Check sheet for the modelled part. Datum: model origin and axes. Units: mm. Face numbers are marked on the shaded views. A direction names the side the tool comes from. Round coordinates to 2 decimals unless told otherwise and drop trailing zeros. Write each loop counter-clockwise with the first axis right and the second up, starting at its lowest first coordinate (ties: lowest second). Pieces come first, ordered by that corner, then holes. Notation, with made-up numbers: (69.5, 4) -> (112.5, 4) arc R25 cw to (112.5, 38) -> close; hole circle Ø7 at (15, 63.5). An arc over 180 degrees is marked (long way). One line per item, written item: value.
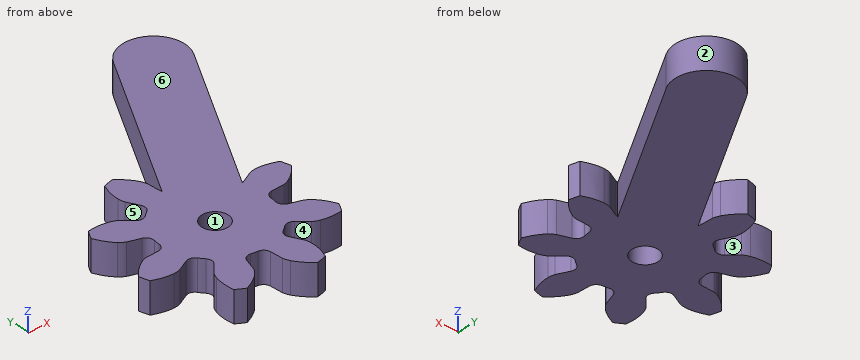
from build123d import *

# Parameters (mm, degrees)
CYLINDER006_R          = 1.7
CYLINDER006_DEPTH      = 10
EXTRUDE011_DEPTH       = 4
EXTRUDE013_DEPTH       = 4
CUT005_PLACEMENT_ANGLE = 30


with BuildPart() as cylinder006:
    # Cylinder006 → Cylinder006 (new body)
    with BuildSketch(Plane(origin=(21, 0, -4), x_dir=(1, 0, 0), z_dir=(0, 0, 1))):
        Circle(CYLINDER006_R)
    extrude(amount=CYLINDER006_DEPTH)


with BuildPart() as extrude011:
    # InvoluteGear004 → Extrude011 (new body)
    with BuildSketch(Plane.XY):
        with BuildLine():
            Line((7.583619, -1.626335), (9.226112, -1.976129))
            add(Edge.make_bspline(
                [(9.226112, -1.976129), (9.323588, -1.988042), (9.615448, -2.006593), (10.112858, -1.891348)],
                knots=[0, 0, 0, 0, 1, 1, 1, 1], degree=3))
            add(Edge.make_bspline(
                [(10.112858, -1.891348), (10.701098, -1.749257), (11.528547, -1.419904), (12.486309, -0.674071)],
                knots=[0, 0, 0, 0, 1, 1, 1, 1], degree=3))
            ThreePointArc((12.486309, -0.674071), (12.504498, 0), (12.486309, 0.674071))
            add(Edge.make_bspline(
                [(12.486309, 0.674071), (11.528547, 1.419904), (10.701098, 1.749257), (10.112858, 1.891348)],
                knots=[0, 0, 0, 0, 1, 1, 1, 1], degree=3))
            add(Edge.make_bspline(
                [(10.112858, 1.891348), (9.615448, 2.006593), (9.323588, 1.988042), (9.226112, 1.976129)],
                knots=[0, 0, 0, 0, 1, 1, 1, 1], degree=3))
            Line((9.226112, 1.976129), (7.583619, 1.626335))
            ThreePointArc((7.583619, 1.626335), (6.928673, 1.725171), (6.502518, 2.232237))
            ThreePointArc((6.502518, 2.232237), (6.351672, 2.630949), (6.176404, 3.019545))
            ThreePointArc((6.176404, 3.019545), (6.119192, 3.679432), (6.512421, 4.212436))
            Line((6.512421, 4.212436), (7.92118, 5.126512))
            add(Edge.make_bspline(
                [(7.92118, 5.126512), (7.99853, 5.187015), (8.218024, 5.380273), (8.488255, 5.813485)],
                knots=[0, 0, 0, 0, 1, 1, 1, 1], degree=3))
            add(Edge.make_bspline(
                [(8.488255, 5.813485), (8.803731, 6.329908), (9.155937, 7.14789), (9.305795, 8.352514)],
                knots=[0, 0, 0, 0, 1, 1, 1, 1], degree=3))
            ThreePointArc((9.305795, 8.352514), (8.842015, 8.842015), (8.352514, 9.305795))
            add(Edge.make_bspline(
                [(8.352514, 9.305795), (7.14789, 9.155937), (6.329908, 8.803731), (5.813485, 8.488255)],
                knots=[0, 0, 0, 0, 1, 1, 1, 1], degree=3))
            add(Edge.make_bspline(
                [(5.813485, 8.488255), (5.380273, 8.218024), (5.187015, 7.99853), (5.126512, 7.92118)],
                knots=[0, 0, 0, 0, 1, 1, 1, 1], degree=3))
            Line((5.126512, 7.92118), (4.212436, 6.512421))
            ThreePointArc((4.212436, 6.512421), (3.679432, 6.119192), (3.019545, 6.176404))
            ThreePointArc((3.019545, 6.176404), (2.630949, 6.351672), (2.232237, 6.502518))
            ThreePointArc((2.232237, 6.502518), (1.725171, 6.928673), (1.626335, 7.583619))
            Line((1.626335, 7.583619), (1.976129, 9.226112))
            add(Edge.make_bspline(
                [(1.976129, 9.226112), (1.988042, 9.323588), (2.006593, 9.615448), (1.891348, 10.112858)],
                knots=[0, 0, 0, 0, 1, 1, 1, 1], degree=3))
            add(Edge.make_bspline(
                [(1.891348, 10.112858), (1.749257, 10.701098), (1.419904, 11.528547), (0.674071, 12.486309)],
                knots=[0, 0, 0, 0, 1, 1, 1, 1], degree=3))
            ThreePointArc((0.674071, 12.486309), (0, 12.504498), (-0.674071, 12.486309))
            add(Edge.make_bspline(
                [(-0.674071, 12.486309), (-1.419904, 11.528547), (-1.749257, 10.701098), (-1.891348, 10.112858)],
                knots=[0, 0, 0, 0, 1, 1, 1, 1], degree=3))
            add(Edge.make_bspline(
                [(-1.891348, 10.112858), (-2.006593, 9.615448), (-1.988042, 9.323588), (-1.976129, 9.226112)],
                knots=[0, 0, 0, 0, 1, 1, 1, 1], degree=3))
            Line((-1.976129, 9.226112), (-1.626335, 7.583619))
            ThreePointArc((-1.626335, 7.583619), (-1.725171, 6.928673), (-2.232237, 6.502518))
            ThreePointArc((-2.232237, 6.502518), (-2.630949, 6.351672), (-3.019545, 6.176404))
            ThreePointArc((-3.019545, 6.176404), (-3.679432, 6.119192), (-4.212436, 6.512421))
            Line((-4.212436, 6.512421), (-5.126512, 7.92118))
            add(Edge.make_bspline(
                [(-5.126512, 7.92118), (-5.187015, 7.99853), (-5.380273, 8.218024), (-5.813485, 8.488255)],
                knots=[0, 0, 0, 0, 1, 1, 1, 1], degree=3))
            add(Edge.make_bspline(
                [(-5.813485, 8.488255), (-6.329908, 8.803731), (-7.14789, 9.155937), (-8.352514, 9.305795)],
                knots=[0, 0, 0, 0, 1, 1, 1, 1], degree=3))
            ThreePointArc((-8.352514, 9.305795), (-8.842015, 8.842015), (-9.305795, 8.352514))
            add(Edge.make_bspline(
                [(-9.305795, 8.352514), (-9.155937, 7.14789), (-8.803731, 6.329908), (-8.488255, 5.813485)],
                knots=[0, 0, 0, 0, 1, 1, 1, 1], degree=3))
            add(Edge.make_bspline(
                [(-8.488255, 5.813485), (-8.218024, 5.380273), (-7.99853, 5.187015), (-7.92118, 5.126512)],
                knots=[0, 0, 0, 0, 1, 1, 1, 1], degree=3))
            Line((-7.92118, 5.126512), (-6.512421, 4.212436))
            ThreePointArc((-6.512421, 4.212436), (-6.119192, 3.679432), (-6.176404, 3.019545))
            ThreePointArc((-6.176404, 3.019545), (-6.351672, 2.630949), (-6.502518, 2.232237))
            ThreePointArc((-6.502518, 2.232237), (-6.928673, 1.725171), (-7.583619, 1.626335))
            Line((-7.583619, 1.626335), (-9.226112, 1.976129))
            add(Edge.make_bspline(
                [(-9.226112, 1.976129), (-9.323588, 1.988042), (-9.615448, 2.006593), (-10.112858, 1.891348)],
                knots=[0, 0, 0, 0, 1, 1, 1, 1], degree=3))
            add(Edge.make_bspline(
                [(-10.112858, 1.891348), (-10.701098, 1.749257), (-11.528547, 1.419904), (-12.486309, 0.674071)],
                knots=[0, 0, 0, 0, 1, 1, 1, 1], degree=3))
            ThreePointArc((-12.486309, 0.674071), (-12.504498, 0), (-12.486309, -0.674071))
            add(Edge.make_bspline(
                [(-12.486309, -0.674071), (-11.528547, -1.419904), (-10.701098, -1.749257), (-10.112858, -1.891348)],
                knots=[0, 0, 0, 0, 1, 1, 1, 1], degree=3))
            add(Edge.make_bspline(
                [(-10.112858, -1.891348), (-9.615448, -2.006593), (-9.323588, -1.988042), (-9.226112, -1.976129)],
                knots=[0, 0, 0, 0, 1, 1, 1, 1], degree=3))
            Line((-9.226112, -1.976129), (-7.583619, -1.626335))
            ThreePointArc((-7.583619, -1.626335), (-6.928673, -1.725171), (-6.502518, -2.232237))
            ThreePointArc((-6.502518, -2.232237), (-6.351672, -2.630949), (-6.176404, -3.019545))
            ThreePointArc((-6.176404, -3.019545), (-6.119192, -3.679432), (-6.512421, -4.212436))
            Line((-6.512421, -4.212436), (-7.92118, -5.126512))
            add(Edge.make_bspline(
                [(-7.92118, -5.126512), (-7.99853, -5.187015), (-8.218024, -5.380273), (-8.488255, -5.813485)],
                knots=[0, 0, 0, 0, 1, 1, 1, 1], degree=3))
            add(Edge.make_bspline(
                [(-8.488255, -5.813485), (-8.803731, -6.329908), (-9.155937, -7.14789), (-9.305795, -8.352514)],
                knots=[0, 0, 0, 0, 1, 1, 1, 1], degree=3))
            ThreePointArc((-9.305795, -8.352514), (-8.842015, -8.842015), (-8.352514, -9.305795))
            add(Edge.make_bspline(
                [(-8.352514, -9.305795), (-7.14789, -9.155937), (-6.329908, -8.803731), (-5.813485, -8.488255)],
                knots=[0, 0, 0, 0, 1, 1, 1, 1], degree=3))
            add(Edge.make_bspline(
                [(-5.813485, -8.488255), (-5.380273, -8.218024), (-5.187015, -7.99853), (-5.126512, -7.92118)],
                knots=[0, 0, 0, 0, 1, 1, 1, 1], degree=3))
            Line((-5.126512, -7.92118), (-4.212436, -6.512421))
            ThreePointArc((-4.212436, -6.512421), (-3.679432, -6.119192), (-3.019545, -6.176404))
            ThreePointArc((-3.019545, -6.176404), (-2.630949, -6.351672), (-2.232237, -6.502518))
            ThreePointArc((-2.232237, -6.502518), (-1.725171, -6.928673), (-1.626335, -7.583619))
            Line((-1.626335, -7.583619), (-1.976129, -9.226112))
            add(Edge.make_bspline(
                [(-1.976129, -9.226112), (-1.988042, -9.323588), (-2.006593, -9.615448), (-1.891348, -10.112858)],
                knots=[0, 0, 0, 0, 1, 1, 1, 1], degree=3))
            add(Edge.make_bspline(
                [(-1.891348, -10.112858), (-1.749257, -10.701098), (-1.419904, -11.528547), (-0.674071, -12.486309)],
                knots=[0, 0, 0, 0, 1, 1, 1, 1], degree=3))
            ThreePointArc((-0.674071, -12.486309), (0, -12.504498), (0.674071, -12.486309))
            add(Edge.make_bspline(
                [(0.674071, -12.486309), (1.419904, -11.528547), (1.749257, -10.701098), (1.891348, -10.112858)],
                knots=[0, 0, 0, 0, 1, 1, 1, 1], degree=3))
            add(Edge.make_bspline(
                [(1.891348, -10.112858), (2.006593, -9.615448), (1.988042, -9.323588), (1.976129, -9.226112)],
                knots=[0, 0, 0, 0, 1, 1, 1, 1], degree=3))
            Line((1.976129, -9.226112), (1.626335, -7.583619))
            ThreePointArc((1.626335, -7.583619), (1.725171, -6.928673), (2.232237, -6.502518))
            ThreePointArc((2.232237, -6.502518), (2.630949, -6.351672), (3.019545, -6.176404))
            ThreePointArc((3.019545, -6.176404), (3.679432, -6.119192), (4.212436, -6.512421))
            Line((4.212436, -6.512421), (5.126512, -7.92118))
            add(Edge.make_bspline(
                [(5.126512, -7.92118), (5.187015, -7.99853), (5.380273, -8.218024), (5.813485, -8.488255)],
                knots=[0, 0, 0, 0, 1, 1, 1, 1], degree=3))
            add(Edge.make_bspline(
                [(5.813485, -8.488255), (6.329908, -8.803731), (7.14789, -9.155937), (8.352514, -9.305795)],
                knots=[0, 0, 0, 0, 1, 1, 1, 1], degree=3))
            ThreePointArc((8.352514, -9.305795), (8.842015, -8.842015), (9.305795, -8.352514))
            add(Edge.make_bspline(
                [(9.305795, -8.352514), (9.155937, -7.14789), (8.803731, -6.329908), (8.488255, -5.813485)],
                knots=[0, 0, 0, 0, 1, 1, 1, 1], degree=3))
            add(Edge.make_bspline(
                [(8.488255, -5.813485), (8.218024, -5.380273), (7.99853, -5.187015), (7.92118, -5.126512)],
                knots=[0, 0, 0, 0, 1, 1, 1, 1], degree=3))
            Line((7.92118, -5.126512), (6.512421, -4.212436))
            ThreePointArc((6.512421, -4.212436), (6.119192, -3.679432), (6.176404, -3.019545))
            ThreePointArc((6.176404, -3.019545), (6.351672, -2.630949), (6.502518, -2.232237))
            ThreePointArc((6.502518, -2.232237), (6.928673, -1.725171), (7.583619, -1.626335))
        make_face()
    extrude(amount=EXTRUDE011_DEPTH)


with BuildPart() as extrude011_1:
    # Extrude011 placement: moved
    add(extrude011.part.moved(Location((21, 0, 0))))


with BuildPart() as cut005:
    # Sketch006 → Extrude013 (new body)
    with BuildSketch(Plane.XY):
        with BuildLine():
            ThreePointArc((-4, 0), (0, -4), (4, 0))
            Line((4, 0), (4, 30))
            ThreePointArc((4, 30), (0, 34), (-4, 30))
            Line((-4, 0), (-4, 30))
        make_face()
    extrude(amount=EXTRUDE013_DEPTH)


with BuildPart() as cut005_1:
    # Extrude013 placement: moved
    add(cut005.part.moved(Location((21, 0, 0))))

    # Fusion003: union Extrude011
    add(extrude011_1.part)

    # Cut005: cut Cylinder006
    add(cylinder006.part, mode=Mode.SUBTRACT)


with BuildPart() as cut005_2:
    # Cut005 placement: moved
    add(cut005_1.part.moved(Location((2.813467, 10.5, 0))).rotate(Axis((2.813467, 10.5, 0), (0, 0, -1)), CUT005_PLACEMENT_ANGLE))


solid = cut005_2.part
Item 1: Material ranges on line 1 along Y through (x, z) = (12, 3.05); line 2 along X through (y, z) = (0, 1); line 3 along Y through (x, z) = (29, 2.25), recorded low to high.
Result set:
line 1: -4.43 to -0.46, 2.91 to 6.89
line 2: 13.97 to 19.3, 22.7 to 28.03
line 3: -6.75 to -2.58, 0.41 to 4.09, 5.86 to 21.86
Item 2: Release check for a two-part mould opening along Y. For the marked faces 1, 2 and 3 record: pulls with the +Y half, pulls with the -Y half, needs draft (parallel to the pull), parting line crosses it, or undercut.
Result set:
face 1: undercut
face 2: parting line crosses it
face 3: pulls with the +Y half
Item 3: Sectioned sample at B-B (y = 18). Enter the section's corners in (x, z).
Result set:
outline: (26.77, 0) -> (36.01, 0) -> (36.01, 4) -> (26.77, 4) -> close
Item 4: Sectioned sample at A-A (x = 36). Enter the section's corners in (y, z), then the cut area to 3 significant figures.
Result set:
outline: (17.98, 0) -> (29.98, 0) -> (29.98, 4) -> (17.98, 4) -> close
area: 48.0 mm^2
Item 5: Depth check by flat-ended pin: pin 1 (1 mm diameter, centred on x = 30.5, z = 0.5, fed in from +Y); pin 2 (2 mm diameter, centred on x = 21, y = 0, fed in from +Z). Enter the tip coordinate at first touch or a pass-through.
Result set:
pin 1: y = 25.32
pin 2: through
Item 6: Tool access check on the marked faces 4, 5 and 6. Record the directions out of +Z, -Z, +X, -X, +Y, -Y that give a thin tool (end or side, any length) a straight path to the whole face; none if there is none.
Result set:
face 4: +Z, -Z, -Y
face 5: +Z, -Z, -X
face 6: +Z, +X, -X, +Y, -Y
